Work out the finished part from the listing and answer in its coordinate system (mm). A direction names the side the tool comes from. Round coordinates to 2 decimals unless told otherwise and drop trailing zeros. Loops run counter-clockwise (first coordinate to the right, second up) from the corner with the lowest first, then second, coordinate; pieces in that order, holes last. Notation, with made-up numbers: (-38, 55.25) -> (-8, 55.25) arc R14 cw to (-8, 67.25) -> close; hole circle Ø1 at (26, -10.5). An arc over 180 degrees is marked (long way). Use one line per item in the form item = value.
Autodesk Inventor part; units mm, degrees
ref_plane "YZ Plane" through (0, 0, 0) normal (1, 0, 0) x (0, 1, 0)
ref_plane "XZ Plane" through (0, 0, 0) normal (0, 1, 0) x (-1, 0, 0)
ref_plane "XY Plane" through (0, 0, 0) normal (0, 0, 1) x (1, 0, 0)
sketch "Sketch1" plane through (0, 0, 0) normal (0, 1, 0) x (-1, 0, 0)
  line L0 (0, 85) -> (0, -85)
  line L1 (25, 0) -> (-25, 0)
  line L2 (0, 85) -> (25, 85)
  line L3 (25, 85) -> (25, -85)
  line L4 (25, -85) -> (-25, -85)
  line L5 (-25, -85) -> (-25, 85)
  line L6 (-25, 85) -> (0, 85)
  point P0 (0, 0)
  point P1 (0, 0)
  point P2 (0, 0)
  dimension "d1" = 50
extrude "Extrusion1" add sketch "Sketch1" along normal blind 63
sketch "Sketch2" plane through (25, 0, 85) normal (1, 0, 0) x (0, 0, -1)
  line L0 (0, 0) -> (170, 0)
  line L1 (170, 0) -> (170, 63)
  line L2 (0, 63) -> (170, 63)
  line L3 (0, 0) -> (0, 63)
  line L4 (0, 0) -> (170, 0)
  line L5 (0, 0) -> (0, 45)
  line L6 (0, 0) -> (0, 63)
  line L7 (0, 45) -> (107, 45)
  line L8 (107, 45) -> (107, 0)
  point P0 (85, 0)
  dimension "d4" = 45
  dimension "d5" = 107
extrude "Extrusion2" cut sketch "Sketch2" against normal up to next contours L3 L7 L8 L0
sketch "Sketch3" plane through (25, 0, -22) normal (0, 0, 1) x (1, 0, 0)
  line L0 (-50, 0) -> (-50, 45)
  line L1 (0, 0) -> (-50, 0)
  line L2 (0, 45) -> (0, 0)
  line L3 (0, 45) -> (-50, 45)
  line L4 (-45, 5) -> (-5, 5)
  line L5 (-5, 30) -> (-5, 5)
  line L6 (-45, 5) -> (-45, 30)
  line L7 (-45, 30) -> (-5, 30)
  point P0 (-25, 0)
  dimension "d10" = 25
  dimension "d11" = 5
  dimension "d12" = 5
  dimension "d13" = 5
extrude "Extrusion3" cut sketch "Sketch3" against normal up to next contours L6 L7 L5 L4
sketch "Sketch4" plane through (25, 0, -85) normal (1, 0, 0) x (0, 0, -1)
  line L0 (-63, 45) -> (-63, 0)
  line L1 (-63, 0) -> (0, 0)
  line L2 (0, 0) -> (0, 63)
  line L3 (-170, 63) -> (0, 63)
  line L4 (-170, 45) -> (-170, 63)
  line L5 (-170, 45) -> (-63, 45)
  line L6 (-170, 45) -> (-165, 45)
  line L7 (-170, 45) -> (-63, 45)
  line L8 (-165, 45) -> (-165, 63)
  line L9 (-170, 63) -> (0, 63)
  line L10 (-170, 45) -> (-170, 53)
  line L11 (-170, 45) -> (-170, 63)
  line L12 (-170, 53) -> (-165, 53)
  line L13 (-170, 53) -> (-170, 63)
  point P0 (-85, 0)
  dimension "d16" = 5
  dimension "d20" = 8
chamfer "Chamfer1" distance 2 angle 45 1 edges at (0, 45, 85)
extrude "Extrusion4" cut sketch "Sketch4" against normal up to next contours L12 L4 L3 L8
chamfer "Chamfer2" distance 5 angle 45 1 edges at (0, 53, 85)
sketch "Sketch5" plane through (25, 0, -85) normal (1, 0, 0) x (0, 0, -1)
  line L0 (-170, 48) -> (-165, 53)
  line L1 (-170, 47) -> (-170, 48)
  line L2 (-168, 45) -> (-170, 47)
  line L3 (-168, 45) -> (-63, 45)
  line L4 (-63, 45) -> (-63, 0)
  line L5 (-63, 0) -> (0, 0)
  line L6 (0, 0) -> (0, 63)
  line L7 (-165, 63) -> (0, 63)
  line L8 (-165, 63) -> (-165, 53)
  line L9 (-165, 53) -> (-165, 63)
  line L10 (-165, 53) -> (-145, 53)
  line L11 (-145, 53) -> (-145, 63)
  point P0 (-85, 0)
  dimension "d26" = 20
extrude "Extrusion5" cut sketch "Sketch5" against normal up to next contours L8 L7 L11 L10
chamfer "Chamfer3" distance 5 angle 45 1 edges at (0, 63, 60)
sketch "Sketch6" plane through (25, 0, -85) normal (1, 0, 0) x (0, 0, -1)
  line L0 (-145, 58) -> (-140, 63)
  line L1 (-145, 58) -> (-145, 53)
  line L2 (-145, 53) -> (-165, 53)
  line L3 (-170, 48) -> (-165, 53)
  line L4 (-170, 47) -> (-170, 48)
  line L5 (-168, 45) -> (-170, 47)
  line L6 (-168, 45) -> (-63, 45)
  line L7 (-63, 45) -> (-63, 0)
  line L8 (-63, 0) -> (0, 0)
  line L9 (0, 0) -> (0, 63)
  line L10 (-140, 63) -> (0, 63)
  line L11 (-170, 47) -> (-170, 0)
  line L12 (-170, 0) -> (-40, 0)
  line L13 (-63, 0) -> (0, 0)
  line L14 (-170, 0) -> (-55, 0)
  line L15 (-55, 0) -> (-55, 45)
  line L16 (-55, 45) -> (0, 45)
  line L17 (0, 0) -> (0, 63)
  line L18 (-55, 45) -> (-55, 53)
  line L19 (-55, 53) -> (0, 53)
  line L20 (-55, 53) -> (-55, 63)
  line L21 (0, 63) -> (-140, 63)
  line L22 (-55, 63) -> (0, 63)
  point P0 (-85, 0)
  dimension "d32" = 130
  dimension "d33" = 115
  dimension "d34" = 8
extrude "Extrusion6" cut sketch "Sketch6" against normal up to next contours L10 L9 L19 L20 | L16 L9 L8 L15
sketch "Sketch7" plane through (25, 53, -30) normal (0, 1, 0) x (1, 0, 0)
  line L0 (-50, 0) -> (-50, 55)
  line L1 (0, 0) -> (-50, 0)
  line L2 (0, 55) -> (0, 0)
  line L3 (-50, 55) -> (0, 55)
  line L4 (0, 0) -> (0, 30)
  line L5 (0, 0) -> (0, 55)
  line L6 (0, 30) -> (-50, 30)
  line L7 (-25, -30) -> (-25, 55)
  circle A0 centre (-25, 30) radius 4
  circle A1 centre (-25, 30) radius 10
  line L8 (0, 0) -> (-15.9346, 34.2212)
  line L9 (-50, 0) -> (-34.0654, 34.2212)
  dimension "d37" = 30
  dimension "d38" = 8
  dimension "d39" = 20
extrude "Extrusion7" cut sketch "Sketch7" against normal up to next contours L0 L6 L9 | L0 L3 L7 A1 L9 L6 | L8 L6 L2 | L3 L2 L6 L8 A1 L7 | A0 L6 L7 | L7 L6 A0 | A0 L7 L6 | L7 A0 L6
chamfer "Chamfer4" distance 5 angle 45 1 edges at (0, 63, -30)
sketch "Sketch8" plane through (0, 63, 0) normal (0, 1, 0) x (1, 0, 0)
  line L0 (-25, -85) -> (25, -85)
  line L1 (-25, 25) -> (25, 25)
  line L2 (-25, 25) -> (-25, -55)
  line L3 (25, -55) -> (-25, -55)
  line L4 (25, -55) -> (25, 25)
  line L5 (25, -85) -> (-25, -85)
  line L6 (25, -85) -> (36, -85)
  line L7 (36, -85) -> (36, -5)
  line L8 (25, -55) -> (25, -30)
  line L9 (25, -55) -> (25, 25)
  line L10 (5, -30) -> (25, -30)
  line L11 (5, -30) -> (5, -12)
  line L12 (5, -12) -> (25, -12)
  line L13 (0, -38) -> (0, 17)
  line L14 (-5, -30) -> (-25, -30)
  line L15 (-5, -30) -> (-5, -12)
  line L16 (-5, -12) -> (-25, -12)
  point P0 (0, 0)
  dimension "d45" = 80
  dimension "d46" = 25
  dimension "d47" = 20
  dimension "d48" = 18
extrude "Extrusion8" cut sketch "Sketch8" against normal blind 10 contours L16 L15 L14 L2 | L4 L10 L11 L12
chamfer "Chamfer5" distance 10 angle 45 1 edges at (15, 63, 12)
chamfer "Chamfer6" distance 10 angle 45 1 edges at (-15, 63, 12)
sketch "Sketch9" plane through (0, 53, 0) normal (0, 1, 0) x (1, 0, 0)
  line L0 (25, -30) -> (5, -30)
  line L1 (25, -12) -> (25, -30)
  line L2 (5, -12) -> (25, -12)
  line L3 (5, -30) -> (5, -12)
  line L4 (-25, -12) -> (-5, -12)
  line L5 (-25, -30) -> (-25, -12)
  line L6 (-5, -30) -> (-25, -30)
  line L7 (-5, -12) -> (-5, -30)
  line L8 (0, 0) -> (0, -34)
  line L9 (25, -12) -> (20, -12)
  line L10 (20, -12) -> (20, -25)
  line L11 (20, -25) -> (25, -25)
  line L12 (25, -83) -> (25, 22)
  line L13 (-5, -12) -> (-25, -12)
  line L14 (-20, -12) -> (-20, -25)
  line L15 (-20, -25) -> (-25, -25)
  dimension "d57" = 5
  dimension "d58" = 13
extrude "Extrusion9" cut sketch "Sketch9" against normal up to next contours L11 L10 L2 L1 | L4 L14 L15 L5
chamfer "Chamfer7" distance 5 angle 45 4 edges at (15, 63, 30) (-15, 63, 30) (25, 49, 25) (-25, 49, 25)
properties part number "PIEZA_3D_1EX"
(1) For faces 4 (the flat face through (20, 18, -26)), 5 (the flat face through (13, 53, 21)), 6 (the flat face through (-15, 60, 32)), 7 (the flat face through (0, 45, 31)), 8 (the flat face through (-20, 49, 18)), determine the directions among +Z, -Z, +X, -X, +Y, -Y from which every point of the face is accessible in a straight line to the end or side of a thin tool.
Completed:
face_4 = +Z, -Z
face_5 = +X, +Y
face_6 = -X, +Y
face_7 = +Z, +X, -X, -Y
face_8 = -X, +Y, -Y
(2) Given P1, Ø6, axis at x = -13, z = -1, coming from the -Y side; P2, Ø9, axis at x = 0, z = -60, coming from the +Y side; P3, Ø2.5, axis at x = -19.5, y = 54.5, coming from the -Z side, each flat-ended and moving along its own axis, determine where each tip first touches the part or whether it passes through.
Completed:
P1 = 45
P2 = 53
P3 = -30
(3) Find section B-B, the plane y = 26.5. Write down the section's boundary in (x, z).
Completed:
outline = (-25, -30) -> (-20, -30) -> (-20, -22) -> (-25, -22) -> close; (20, -30) -> (25, -30) -> (25, -22) -> (20, -22) -> close
(4) For a pull along X with two mould halves and no side action, classify faces 1 (the flat face through (0, 30, -26)), 2 (the flat face through (-13, 53, 21)), 3 (the flat face through (-5, 58, 19)) as +X half, -X half, draft (parallel to the pull), parting line (faces both ways), or undercut.
Completed:
face_1 = undercut
face_2 = draft
face_3 = -X half
(5) Consider L1, parallel to Y at x = 9.5, z = 42.5; L2, parallel to X at y = 15, z = -25.5; L3, parallel to Y at x = 15, z = -39.5. Determine where each line is inside the solid, lowest interval first.
Completed:
L1 = 45 to 63
L2 = -25 to -20, 20 to 25
L3 = 45 to 53
(6) Find section A-A, the plane x = 0. Write down the section's boundary in (y, z), then the cut area to 3 significant figures.
Completed:
outline = (0, -30) -> (5, -30) -> (5, -22) -> (0, -22) -> close; (30, -30) -> (45, -30) -> (45, -56) -> (53, -56) -> (53, -30) -> (58, -30) -> (63, -25) -> (63, 55) -> (58, 60) -> (53, 60) -> (53, 80) -> (48, 85) -> (47, 85) -> (45, 83) -> (45, -22) -> (30, -22) -> close; (45, -70) -> (53, -70) -> (53, -64) -> (45, -64) -> close
area = 2,200 mm2
(7) Find section C-C, the plane z = -60. Write down the section's boundary in (x, y).
Completed:
outline = (-11.03, 45) -> (-4, 45) -> (-4, 53) -> (-11.03, 53) -> close; (4, 45) -> (11.03, 45) -> (11.03, 53) -> (4, 53) -> close
(8) Find section D-D, the plane y = 59.5. Write down the section's boundary in (x, z), then the cut area to 3 significant figures.
Completed:
outline = (-25, -28.5) -> (25, -28.5) -> (25, 5.5) -> (5, 5.5) -> (5, 31.5) -> (25, 31.5) -> (25, 58.5) -> (-25, 58.5) -> (-25, 31.5) -> (-5, 31.5) -> (-5, 5.5) -> (-25, 5.5) -> close
area = 3,310 mm2
